Check sheet for the modelled part. Datum: model origin and axes. Units: mm. Face numbers are marked on the shaded views. A direction names the side the tool comes from. Give positions to 0.01 mm unless a question says otherwise; leave off trailing zeros. Loops run counter-clockwise (first coordinate to the right, second up) from the corner with the lowest first, then second, coordinate; pieces in that order, holes last. Notation, with made-up numbers: M 44.5,75.25 L 72.5,75.25 A11 cw 72.5,87.25 Z; hole C 7.25,-7.5 d10. An arc over 180 degrees is marked long. Put each result on its own line as item: value. Start each with the question number.
```python
from build123d import *

# Parameters (mm, degrees)
SKETCH1_R                   = 150
BOSS_EXTRUDE1_DEPTH         = 75
CHAMFER1_SIZE               = 10
BOSS_EXTRUDE2_START         = -75
BOSS_EXTRUDE2_DEPTH         = 10
CHAMFER2_SIZE               = 7
BOSS_EXTRUDE3_DEPTH         = 10
SKETCH4_R                   = 4
CUT_EXTRUDE1_DEPTH          = 255.641782801
CIRPATTERN1_COUNT           = 4
CIRPATTERN1_COPY_1_DEPTH    = 10
CIRPATTERN1_COPY_2_DEPTH    = 10
CIRPATTERN1_COPY_3_DEPTH    = 10
CIRPATTERN1_COPY_4_SKETCH_R = 4
CIRPATTERN1_COPY_4_DEPTH    = 255.641782801
CIRPATTERN1_COPY_5_SKETCH_R = 4
CIRPATTERN1_COPY_5_DEPTH    = 255.641782801
CIRPATTERN1_COPY_6_SKETCH_R = 4
CIRPATTERN1_COPY_6_DEPTH    = 255.641782801
CUT_EXTRUDE2_START          = -60
CUT_EXTRUDE2_DEPTH          = 347.111647957
CIRPATTERN2_COUNT           = 4
SKETCH6_R                   = 110
BOSS_EXTRUDE4_DEPTH         = 9
BOSS_EXTRUDE4_TAPER         = 45
SKETCH7_R                   = 10
BOSS_EXTRUDE5_DEPTH         = 20
L_EK1_SCALE                 = 0.2


with BuildPart() as part:
    # Sketch1 → Boss-Extrude1 (new body)
    with BuildSketch(Plane(origin=(0, 0, 0), x_dir=(1, 0, 0), z_dir=(0, 1, 0))):
        with Locations(Location((0, 0, 0), (0, 0, 270))):
            Circle(SKETCH1_R)
    extrude(amount=BOSS_EXTRUDE1_DEPTH)

    # Chamfer1
    chamfer1_edges = [part.edges().sort_by_distance(p)[0] for p in [
        (0, 75, -150),
    ]]
    chamfer(chamfer1_edges, length=CHAMFER1_SIZE)

    # Sketch2 → Boss-Extrude2 (add)
    with BuildSketch(Plane(origin=(0, 75, 0), x_dir=(1, 0, 0), z_dir=(0, 1, 0)).offset(BOSS_EXTRUDE2_START)):
        with BuildLine():
            Line((-195.236875483, 37.5), (-195.236875483, -37.5))
            Line((-195.236875483, -37.5), (-145.236875483, -37.5))
            ThreePointArc((-145.236875483, -37.5), (-150, 0), (-145.236875483, 37.5))
            Line((-145.236875483, 37.5), (-195.236875483, 37.5))
        make_face()
    boss_extrude2 = extrude(amount=BOSS_EXTRUDE2_DEPTH)

    # Chamfer2
    chamfer2_edges = [part.edges().sort_by_distance(p)[0] for p in [
        (-195.236875483, 5, 37.5),
        (-195.236875483, 5, -37.5),
    ]]
    chamfer(chamfer2_edges, length=CHAMFER2_SIZE)

    # Sketch3 → Boss-Extrude3 (add)
    with BuildSketch(Plane.XY.offset(37.5)):
        Polygon((-150, 65), (-170.556875483, 65), (-188.236875483, 10), (-188.236875483, 0), (-145.236875483, 0), (-145.236875483, 65), align=None)
    boss_extrude3 = extrude(amount=-BOSS_EXTRUDE3_DEPTH)

    # Sketch4 → Cut-Extrude1 (cut, symmetric)
    with BuildSketch(Plane(origin=(0, 10, 0), x_dir=(1, 0, 0), z_dir=(0, 1, 0))):
        with Locations(Location((-172.618437741, -13.75, 0), (0, 0, 270))):
            Circle(SKETCH4_R)
    cut_extrude1 = extrude(amount=CUT_EXTRUDE1_DEPTH, both=True, mode=Mode.SUBTRACT)

    # Mirror1: Boss-Extrude3, Cut-Extrude1 across plane
    add(boss_extrude3.mirror(Plane.XY))
    add(cut_extrude1.mirror(Plane.XY), mode=Mode.SUBTRACT)

    # CirPattern1: Boss-Extrude2, Boss-Extrude3, Cut-Extrude1 ×4 about axis
    cirpattern1_axis = Axis((0, 0, 0), (0, 1, 0))
    add([boss_extrude2.rotate(cirpattern1_axis, i * 360 / CIRPATTERN1_COUNT) for i in range(1, CIRPATTERN1_COUNT)])
    add([boss_extrude3.rotate(cirpattern1_axis, i * 360 / CIRPATTERN1_COUNT) for i in range(1, CIRPATTERN1_COUNT)])
    add([cut_extrude1.rotate(cirpattern1_axis, i * 360 / CIRPATTERN1_COUNT) for i in range(1, CIRPATTERN1_COUNT)], mode=Mode.SUBTRACT)

    # CirPattern1 copy 1 sketch → CirPattern1 copy 1 (add)
    with BuildSketch(Plane(origin=(-37.5, 0, 0), x_dir=(0, 0, -1), z_dir=(-1, 0, 0))):
        Polygon((-150, -65), (-170.556875483, -65), (-188.236875483, -10), (-188.236875483, 0), (-145.236875483, 0), (-145.236875483, -65), align=None)
    extrude(amount=-CIRPATTERN1_COPY_1_DEPTH)

    # CirPattern1 copy 2 sketch → CirPattern1 copy 2 (add)
    with BuildSketch(Plane(origin=(0, 0, 37.5), x_dir=(-1, 0, 0), z_dir=(0, 0, 1))):
        Polygon((-150, -65), (-170.556875483, -65), (-188.236875483, -10), (-188.236875483, 0), (-145.236875483, 0), (-145.236875483, -65), align=None)
    extrude(amount=-CIRPATTERN1_COPY_2_DEPTH)

    # CirPattern1 copy 3 sketch → CirPattern1 copy 3 (add)
    with BuildSketch(Plane(origin=(37.5, 0, 0), x_dir=(0, 0, 1), z_dir=(1, 0, 0))):
        Polygon((-150, -65), (-170.556875483, -65), (-188.236875483, -10), (-188.236875483, 0), (-145.236875483, 0), (-145.236875483, -65), align=None)
    extrude(amount=-CIRPATTERN1_COPY_3_DEPTH)

    # CirPattern1 copy 4 sketch → CirPattern1 copy 4 (cut, symmetric)
    with BuildSketch(Plane(origin=(0, 10, 0), x_dir=(0, 0, -1), z_dir=(0, 1, 0))):
        with Locations((-172.618437741, 13.75)):
            Circle(CIRPATTERN1_COPY_4_SKETCH_R)
    extrude(amount=CIRPATTERN1_COPY_4_DEPTH, both=True, mode=Mode.SUBTRACT)

    # CirPattern1 copy 5 sketch → CirPattern1 copy 5 (cut, symmetric)
    with BuildSketch(Plane(origin=(0, 10, 0), x_dir=(-1, 0, 0), z_dir=(0, 1, 0))):
        with Locations((-172.618437741, 13.75)):
            Circle(CIRPATTERN1_COPY_5_SKETCH_R)
    extrude(amount=CIRPATTERN1_COPY_5_DEPTH, both=True, mode=Mode.SUBTRACT)

    # CirPattern1 copy 6 sketch → CirPattern1 copy 6 (cut, symmetric)
    with BuildSketch(Plane.ZX.offset(10)):
        with Locations((-172.618437741, 13.75)):
            Circle(CIRPATTERN1_COPY_6_SKETCH_R)
    extrude(amount=CIRPATTERN1_COPY_6_DEPTH, both=True, mode=Mode.SUBTRACT)

    # Sketch5 → Cut-Extrude2 (cut)
    with BuildSketch(Plane(origin=(0, 75, 0), x_dir=(1, 0, 0), z_dir=(0, 1, 0)).offset(CUT_EXTRUDE2_START)):
        with BuildLine():
            Line((-112.583302492, -65), (-129.903810568, -75))
            ThreePointArc((-129.903810568, -75), (-106.066017178, -106.066017178), (-75, -129.903810568))
            Line((-75, -129.903810568), (-65, -112.583302492))
            ThreePointArc((-65, -112.583302492), (-91.923881554, -91.923881554), (-112.583302492, -65))
        make_face()
    cut_extrude2 = extrude(amount=CUT_EXTRUDE2_DEPTH, mode=Mode.SUBTRACT)

    # CirPattern2: Cut-Extrude2 ×4 about axis
    cirpattern2_axis = Axis((0, 75, 0), (0, -1, 0))
    for i in range(1, CIRPATTERN2_COUNT):
        add(cut_extrude2.rotate(cirpattern2_axis, i * 360 / CIRPATTERN2_COUNT), mode=Mode.SUBTRACT)

    # Sketch6 → Boss-Extrude4 (add)
    with BuildSketch(Plane(origin=(0, 75, 0), x_dir=(1, 0, 0), z_dir=(0, 1, 0))):
        Circle(SKETCH6_R)
    extrude(amount=BOSS_EXTRUDE4_DEPTH, taper=BOSS_EXTRUDE4_TAPER)

    # Sketch7 → Boss-Extrude5 (add)
    with BuildSketch(Plane(origin=(0, 84, 0), x_dir=(1, 0, 0), z_dir=(0, 1, 0))):
        with Locations(Location((0, 0, 0), (0, 0, 270))):
            Circle(SKETCH7_R)
    extrude(amount=BOSS_EXTRUDE5_DEPTH)


with BuildPart() as part_1:
    # Ölçek1: scaled about (0.0171202, 38.41973145, 0)
    add(part.part.scale(L_EK1_SCALE).moved(Location((0.01369616, 30.73578516, 0))))


solid = part_1.part
```
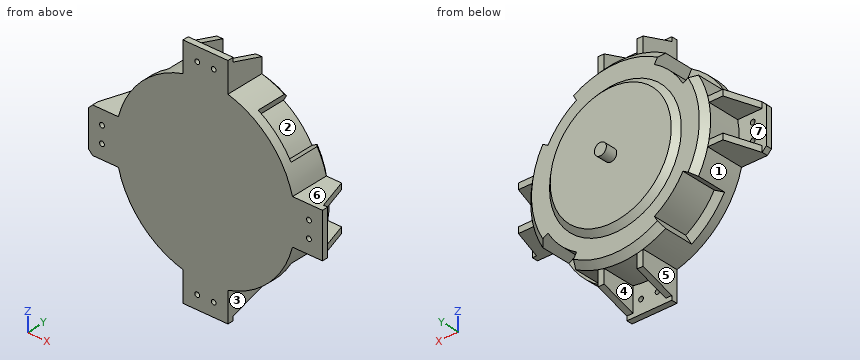
Q1. Access from +Z, -Z, +X, -X, +Y, -Y to the whole of each face (thin tool, end or side, straight path). Record for the marked faces 4, 5, 6 and 7.
Q2. Mould release check, pull along Z, two halves, no side actions. Record for the marked faces 1, 2 and 3: pulls with the +Z half, pulls with the -Z half, needs draft (parallel to the pull), parting line crosses it, or undercut.
Q3. Thickness scan on line 1 along X through (y, z) = (41.25, 14); line 2 along Z through (x, y) = (-14, 40); line 3 along X through (y, z) = (33.25, 32). Record the ranges inside material, lowest first. Write a range as [from, to].
Q4. Section check A-A, the plane y = 50. Record the cut outline in (x, z).
Q5. Depth check by flat-ended pin: P1, Ø1.5, axis at y = 41.5, z = 7.5, coming from the -X side; P2, Ø6.5, axis at x = 33, y = 41, coming from the -Z side; P3, Ø6.5, axis at x = -22, z = -21.5, coming from the +Y side; P4, Ø2, axis at x = -2.74, z = 34.52, coming from the -Y side. Enter the tip coordinate at first touch or a pass-through.
Found:
1. face 4: -Z, +Y
1. face 5: -Z, -X, +Y, -Y
1. face 6: +Z, +X, +Y, -Y
1. face 7: -X, +Y
2. face 1: pulls with the -Z half
2. face 2: undercut
2. face 3: needs draft
3. line 1: x = [-26.52, -24.24], [-21.9, 21.92], [24.26, 26.55]
3. line 2: z = [-26.53, -24.27], [-21.9, 21.9], [24.27, 26.53]
3. line 3: x = [-7.49, -5.49], [5.51, 7.51]
4. outline: C 0.01,0 d4
5. P1: stops at x = -35.06
5. P2: stops at z = -7.5
5. P3: stops at y = 33.74
5. P4: stops at y = 30.74
